Verification items for this drawing (mm, ordinates from the low corner). A direction names the side the tool comes from. Coordinates: 2 decimals unless noted, no trailing zeros. Order: outer loops, then holes, each group sorted by start corner. A loop starts at its lowest first (then second) coordinate and runs counter-clockwise, first axis right, second up. Notation, with made-up numbers: M 85,19.25 L 134,19.25 A21 cw 134,57.25 Z; hole C 8.25,82.25 d4. An arc over 180 degrees is marked long. Answer as a JSON object with one key per item and string values. Group by question number.
(1) Gauge pin test, flat ends, axial feed: pin 1 Ø4 at (x, y) = (3.5, 33.5) entering from +Z; pin 2 Ø3 at (x, y) = (4, 54) entering from -Z. Record the tip position at first contact, or that the pin passes through.
(2) Cross-section at B-B (x = 4). Count the separate pieces of the cut face and the enclosed holes in it, plus the area to 3 significant figures.
(3) Cross-section at C-C (y = 54). Enter the section's corners in (x, z), plus the area to 3 significant figures.
(4) Mould release check, pull along Y, two halves, no side actions. Record for the marked faces 3, 4 and 5: released by +Y, released by -Y, zero draft, split by the parting line, or undercut.
(5) Access from +Z, -Z, +X, -X, +Y, -Y to the whole of each face (thin tool, end or side, straight path). Record for the marked faces 1 and 2.
(6) Cross-section at D-D (y = 33.5). Enter the section's corners in (x, z), plus the area to 3 significant figures.
(7) Material ranges on line 1 (Y direction, x = 4, z = 28.6); line 2 (Y direction, x = 4, z = 7); line 3 (Y direction, x = 4.75, z = 25.5), recorded low to high.
(8) Cross-section at A-A (z = 12). Enter the section's corners in (x, y).
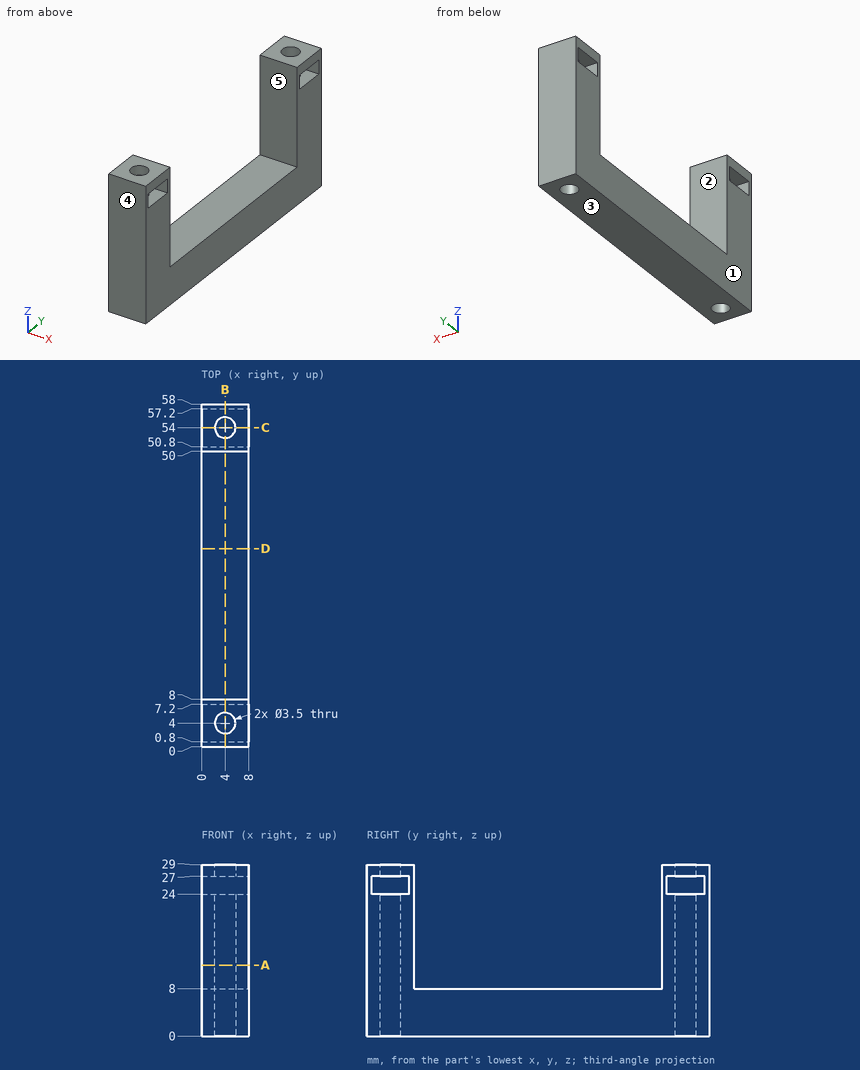
Taken from the geometry:
{
 "1": {"pin 1": "stops at z = 8", "pin 2": "passes through"},
 "2": {"separate pieces": "3", "enclosed holes": "0", "area": "580 mm²"},
 "3": {"outline": "M 0,0 L 2.25,0 L 2.25,24 L 0,24 Z; M 0,27 L 2.25,27 L 2.25,29 L 0,29 Z; M 5.75,0 L 8,0 L 8,24 L 5.75,24 Z; M 5.75,27 L 8,27 L 8,29 L 5.75,29 Z", "area": "117 mm²"},
 "4": {"face 3": "zero draft", "face 4": "released by -Y", "face 5": "undercut"},
 "5": {"face 1": "+Z, -Z, -X, +Y, -Y", "face 2": "+Z, +X, -X"},
 "6": {"outline": "M 0,0 L 8,0 L 8,8 L 0,8 Z", "area": "64.0 mm²"},
 "7": {"line 1": "y = 0 to 2.25, 5.75 to 8, 50 to 52.25, 55.75 to 58", "line 2": "y = 0 to 2.25, 5.75 to 52.25, 55.75 to 58", "line 3": "y = 0 to 0.8, 7.2 to 8, 50 to 50.8, 57.2 to 58"},
 "8": {"outline": "M 0,0 L 8,0 L 8,8 L 0,8 Z; M 0,50 L 8,50 L 8,58 L 0,58 Z; hole C 4,4 d3.5; hole C 4,54 d3.5"}
}
